from build123d import *

# Parameters (mm, degrees)
F0_W     = 66.04
F0_H     = 43.139034
F1_DEPTH = 2.54
F2_W     = 18.795862
F2_H     = 35.368388
F3_DEPTH = 25.4
F4_W     = 17.531056
F4_H     = 35.368388
F5_DEPTH = 25.4
F6_R     = 7.770645
F7_DEPTH = 2.54
F8_R     = 4.163339
F9_DEPTH = 25.4


with BuildPart() as f1:
    # F0 (on Top) → F1 (new body)
    with BuildSketch(Plane.XY):
        with Locations((-0.843987, -0.339514)):
            Rectangle(F0_W, F0_H)
    extrude(amount=F1_DEPTH)

    # F2 (on face) → F3 (cut)
    with BuildSketch(Plane.XY.offset(2.54)):
        with Locations((12.255906, -4.224837)):
            Rectangle(F2_W, F2_H)
    extrude(amount=-F3_DEPTH, mode=Mode.SUBTRACT)

    # F4 (on face) → F5 (cut)
    with BuildSketch(Plane.XY.offset(2.54)):
        with Locations((-15.148921, -4.224837)):
            Rectangle(F4_W, F4_H)
    extrude(amount=-F5_DEPTH, mode=Mode.SUBTRACT)

    # F6 (on face) → F7 (join)
    with BuildSketch(Plane.XY.offset(2.54)):
        with Locations((32.176013, 21.230003)):
            Circle(F6_R)
    extrude(amount=-F7_DEPTH)

    # F8 (on face) → F9 (cut)
    with BuildSketch(Plane.XY.offset(2.54)):
        with Locations((32.176013, 21.230003)):
            Circle(F8_R)
    extrude(amount=-F9_DEPTH, mode=Mode.SUBTRACT)


solid = f1.part
Source: CAD feature listing. Evaluate the final solid. Frame: model axes, mm. A direction names the side the tool comes from. Coordinates: 2 decimals unless noted, no trailing zeros. Order: outer loops, then holes, each group sorted by start corner. A loop starts at its lowest first (then second) coordinate and runs counter-clockwise, first axis right, second up. Notation, with made-up numbers: M 59.5,52.5 L 92.5,52.5 A35 cw 92.5,90.5 Z; hole C 87,79 d2. An arc over 180 degrees is marked long. Write each question's results on one line, items separated by ' | '. Start each with the question number.
1. Section C-C, the plane x = 29.5. Return the cut outline in (y, z).
2. Section D-D, the plane y = 22. Return the cut outline in (x, z).
3. Reachability of faces 4 (the face through (-5, 21.23, 1)), 5 (the face through (-15, 13.459, 1)), 6 (the face through (32.176, -4, 1)), 7 (the face through (-2, -21.909, 1)), 8 (the face through (-33.864, -1, 1)) from +Z, -Z, +X, -X, +Y, -Y: full face, straight path, thin tool, end or side. Return the list, or none.
4. Section B-B, the plane z = 0.95. Return the cut outline in (x, y).
5. Material intervals for L1, parallel to X at y = -1, z = 1; L2, parallel to Y at x = 34.5, z = 1.15; L3, parallel to Y at x = 10.5, z = 1.4, sorted ascending.
6. Pin query (flat end, axial travel): pin 1 (0.8 mm diameter, centred on y = -7.5, z = 1, fed in from +X); pin 2 (4 mm diameter, centred on x = -18.5, y = 9.5, fed in from +Z); pin 3 (0.8 mm diameter, centred on x = 10.5, z = 1.5, fed in from -Y); pin 4 (1 mm diameter, centred on x = -14.5, z = 1, fed in from +Y). Return the tip coordinate at first contact, or that it passes through.
7. Section A-A, the plane y = -4. Return the cut outline in (x, z), then the cut area to 3 significant figures.
8. Draft query along Y for faces 1 (the face through (2.5, 3.9, 0)), 2 (the face through (-29, -21.909, 1)), 3 (the face through (28.017, 21.413, 1.288)). Return one class per face: +Y half, -Y half, draft (parallel to the pull), parting line (faces both ways), or undercut.
Solution:
1) outline: M -21.91,0 L 18.04,0 L 18.04,2.54 L -21.91,2.54 Z; M 24.42,0 L 28.53,0 L 28.53,2.54 L 24.42,2.54 Z
2) outline: M 24.44,0 L 28.08,0 L 28.08,2.54 L 24.44,2.54 Z; M 36.27,0 L 39.91,0 L 39.91,2.54 L 36.27,2.54 Z
3) face 4: +Z, -Z, -X, +Y | face 5: +Z, -Z, -Y | face 6: +Z, -Z, +X, -Y | face 7: +Z, -Z, +X, -X, -Y | face 8: +Z, -Z, -X, +Y, -Y
4) outline: M -33.86,-21.91 L -23.91,-21.91 L -23.91,13.46 L -6.38,13.46 L -6.38,-21.91 L 2.86,-21.91 L 2.86,13.46 L 21.65,13.46 L 21.65,-21.91 L 32.18,-21.91 L 32.18,13.46 A7.77 ccw long 24.41,21.23 L -33.86,21.23 Z; hole C 32.18,21.23 d8.33
5) L1: -33.86 to -23.91, -6.38 to 2.86, 21.65 to 32.18 | L2: 13.82 to 17.78, 24.68 to 28.64 | L3: 13.46 to 21.23
6) pin 1: x = 32.18 | pin 2: through | pin 3: y = 13.46 | pin 4: y = 21.23
7) outline: M -33.86,0 L -23.91,0 L -23.91,2.54 L -33.86,2.54 Z; M -6.38,0 L 2.86,0 L 2.86,2.54 L -6.38,2.54 Z; M 21.65,0 L 32.18,0 L 32.18,2.54 L 21.65,2.54 Z | area: 75.5 mm²
8) face 1: draft | face 2: -Y half | face 3: undercut
